Can you work these out from the model? Positions are in its coordinate system, mm. Face numbers are marked on the shaded views. A direction names the side the tool comes from. Give positions to 0.01 mm unless a question says otherwise; leave off trailing zeros. Loops run counter-clockwise (first coordinate to the right, second up) from the corner with the lowest first, then second, coordinate; pieces in that order, holes last. Notation, with made-up numbers: M -9.5,0.5 L 20.5,0.5 A33 cw 20.5,36.5 Z; hole C -2.5,-29.75 d3. An arc over 180 degrees is marked long. Answer as a JSON object with one key per item and string values.
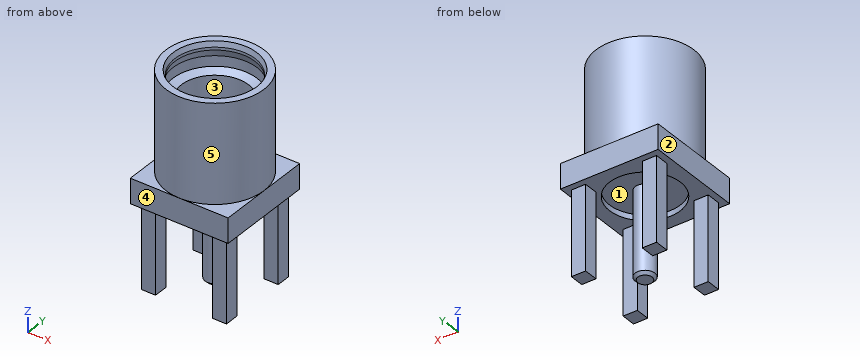
```python
from build123d import *

# Parameters (mm, degrees)
SKETCH_W           = 3.51
SKETCH_H           = 3.51
PAD_DEPTH          = 0.89
SKETCH003_R        = 0.355
PAD002_DEPTH       = 2.91
PAD003_DEPTH       = 1.46
SKETCH005_R        = 1.27
SKETCH005_R_2      = 0.355
POCKET_DEPTH       = 0.2
SKETCH002_W        = 0.51
SKETCH002_H        = 0.51
PAD005_DEPTH       = 3.02
POLARPATTERN_COUNT = 4
CHAMFER_SIZE       = 0.1


with BuildPart() as part:
    # Sketch → Pad (new body)
    with BuildSketch(Plane.XY):
        Rectangle(SKETCH_W, SKETCH_H)
    extrude(amount=PAD_DEPTH)

    # Sketch001 → Revolution (revolve)
    with BuildSketch(Plane.XZ):
        Polygon((1.755, 0.89), (0.825, 0.89), (0.825, 1.82), (1.205, 1.82), (1.205, 3.42), (1.505, 3.53), (1.505, 3.9), (1.44, 4.14), (1.44, 4.24), (1.505, 4.42), (1.755, 4.42), align=None)
    revolve(axis=Axis((0, 0, 0), (0, 0, 1)))

    # Sketch003 → Pad002 (join)
    with BuildSketch(Plane(origin=(0, 0, 0), x_dir=(1, 0, 0), z_dir=(0, 0, -1))):
        Circle(SKETCH003_R)
    extrude(amount=PAD002_DEPTH)

    # Sketch004 → Pad003 (join)
    with BuildSketch(Plane.XY.offset(0.89)):
        with BuildLine():
            ThreePointArc((0.188746, 0.08), (0, 0.205), (-0.188746, 0.08))
            Line((-0.345868, 0.08), (-0.188746, 0.08))
            ThreePointArc((0.345868, 0.08), (0, 0.355), (-0.345868, 0.08))
            Line((0.188746, 0.08), (0.345868, 0.08))
        make_face()
        with BuildLine():
            ThreePointArc((-0.188746, -0.08), (0, -0.205), (0.188746, -0.08))
            Line((0.188746, -0.08), (0.345868, -0.08))
            ThreePointArc((-0.345868, -0.08), (0, -0.355), (0.345868, -0.08))
            Line((-0.345868, -0.08), (-0.188746, -0.08))
        make_face()
    extrude(amount=PAD003_DEPTH)

    # Sketch005 (on Face3 of Pad003) → Pocket (cut)
    with BuildSketch(Plane(origin=(0, 0, 0), x_dir=(1, 0, 0), z_dir=(0, 0, -1))):
        Circle(SKETCH005_R)
        Circle(SKETCH005_R_2, mode=Mode.SUBTRACT)
    extrude(amount=-POCKET_DEPTH, mode=Mode.SUBTRACT)

    # Sketch002 (on Face1 of Revolution) → Pad005 (join)
    with BuildSketch(Plane(origin=(0, 0, 0), x_dir=(1, 0, 0), z_dir=(0, 0, -1))):
        with Locations((-1.27, 1.273)):
            Rectangle(SKETCH002_W, SKETCH002_H)
    pad005 = extrude(amount=PAD005_DEPTH)

    # PolarPattern: Pad005 ×4 about axis
    polarpattern_axis = Axis((0, 0, 0), (0, 0, -1))
    for i in range(1, POLARPATTERN_COUNT):
        add(pad005.rotate(polarpattern_axis, i * 360 / POLARPATTERN_COUNT))

    # Chamfer
    chamfer_edges = [part.edges().sort_by_distance(p)[0] for p in [
        (-0.355, 0, -2.91),
    ]]
    chamfer(chamfer_edges, length=CHAMFER_SIZE)


solid = part.part
```
1) Suppose I cut it at C-C, the plane z = 4. Write out the boundary of the cut face in (x, y) (3 decimals).
Answer list:
{"outline": "C 0,0 d3.51; hole C 0,0 d2.956"}
2) Will these pins go through, and if not, where does the flat tip stop? pin 1 Ø2 at (x, y) = (0, 0) entering from -Z; pin 2 Ø1.3 at (x, y) = (0, 0) entering from +Z; pin 3 Ø2 at (x, y) = (0.5, -0.5) entering from -Z; pin 4 Ø0.6 at (y, z) = (1.5, -1.5) entering from -X.
Answer list:
{"pin 1": "z = -2.91", "pin 2": "z = 2.35", "pin 3": "z = -3.02", "pin 4": "x = -1.53"}
3) Suppose I cut it at A-A, the plane z = 1.5. Write out the boundary of the cut face in (x, y) (3 decimals).
Answer list:
{"outline": "C 0,0 d3.51; M -0.346,-0.08 A0.355 ccw 0.346,-0.08 L 0.189,-0.08 A0.205 cw -0.189,-0.08 Z; M -0.346,0.08 L -0.189,0.08 A0.205 cw 0.189,0.08 L 0.346,0.08 A0.355 ccw Z; hole C 0,0 d1.65"}
4) Suppose I cut it at B-B, the plane z = -0.75. Write out the boundary of the cut face in (x, y) (3 decimals).
Answer list:
{"outline": "M -1.528,1.015 L -1.018,1.015 L -1.018,1.525 L -1.528,1.525 Z; M -1.525,-1.528 L -1.015,-1.528 L -1.015,-1.018 L -1.525,-1.018 Z; C 0,0 d0.71; M 1.015,1.018 L 1.525,1.018 L 1.525,1.528 L 1.015,1.528 Z; M 1.018,-1.525 L 1.528,-1.525 L 1.528,-1.015 L 1.018,-1.015 Z"}
5) If we mould it in two halves opening along Y, with no side actions, what happens to the marked faces 3, 4 and 5? For each: +Y half, -Y half, draft (parallel to the pull), parting line (faces both ways), or undercut.
Answer list:
{"face 3": "undercut", "face 4": "-Y half", "face 5": "parting line"}
6) Please list where these lines run through material, in increasing order: line 1 along X through (y, z) = (0, 0.15) (3 decimals); line 2 along Y through (x, z) = (0, 3.8) (3 decimals); line 3 along Y through (x, z) = (0, 4.2) (3 decimals). Write a range as from..to.
Answer list:
{"line 1": "-1.755..-1.27, -0.355..0.355, 1.27..1.755", "line 2": "-1.755..-1.505, 1.505..1.755", "line 3": "-1.755..-1.44, 1.44..1.755"}
7) For the marked faces 1 and 2, which set-ups out of +Z, -Z, +X, -X, +Y, -Y let a thin tool reach every point of the face, with its end or its side?
Answer list:
{"face 1": "-Z", "face 2": "+Z, -Z, -X, +Y, -Y"}
